For this review, take the finished solid that the model builds, in its own axes (mm). A direction names the side the tool comes from. Give positions to 0.01 mm unless a question says otherwise; leave off trailing zeros. Order: outer loops, then holes, each group sorted by start corner. A loop starts at its lowest first (then second) coordinate and runs counter-clockwise, first axis right, second up. Notation, with made-up numbers: (30.5, 9.25) - (62.5, 9.25) arc R23 ccw to (62.5, 18.25) - close; hole circle Ø2 at (37.25, 19.25). An arc over 180 degrees is marked (long way). Use a Markdown table: item, result. Add a question column.
1) Mouldability with a two-part tool opening along X and no side actions: class faces 3 (the face through (0, 0, 0)), 4 (the face through (9.954, 11.671, 2.504)), 5 (the face through (-2.88, 21.91, 2.5)) as released by +X, released by -X, zero draft, split by the parting line, or undercut.
2) We need section C-C on z = 63.5. Write out the cut boundary in (x, y), then the cut area to 3 significant figures.
3) Clearance check with flat-ended pins moving along their axes: P1, Ø2, axis at x = -9, z = 37.5, coming from the +Y side; P2, Ø10, axis at x = 12.89, y = -12.89, coming from the +Z side; P3, Ø3, axis at y = -7, z = 50.5, coming from the +X side. State where each tip first meets the part, or that it passes through.
4) Wall thickness on L1, parallel to Z at x = 6, y = -15; L2, parallel to Z at x = -11, y = 3.5; L3, parallel to Y at x = -5, z = 59: over which ranges is each line inside the solid? List them lowest first.
5) We need section A-A on x = 0. Write out the cut boundary in (y, z), then the cut area to 3 significant figures.
6) Machinability: for faces 1 (the face through (13.84, -9.86, 2.5)), 2 (the face through (1.93, 8.68, 67.47)), which of the approach directions +Z, -Z, +X, -X, +Y, -Y give a long, thin tool a straight path to every point of the face, cutting with its end or side? Answer none if there is none.
7) We need section D-D on z = 34. Write out the cut boundary in (x, y), then the cut area to 3 significant figures.
```python
from build123d import *

# Parameters (mm, degrees)
SKETCH1_R           = 22.098
BOSS_EXTRUDE1_DEPTH = 5.08
SKETCH2_R           = 14.351
BOSS_EXTRUDE2_DEPTH = 38.1
SKETCH3_R           = 11.811
BOSS_EXTRUDE3_DEPTH = 17.78
SKETCH4_R           = 8.89
BOSS_EXTRUDE4_DEPTH = 13.208
SKETCH6_R           = 3.175
CUT_EXTRUDE1_DEPTH  = 5.08
CIRPATTERN1_COUNT   = 4


with BuildPart() as part:
    # Sketch1 → Boss-Extrude1 (new body)
    with BuildSketch(Plane.XY):
        Circle(SKETCH1_R)
    extrude(amount=BOSS_EXTRUDE1_DEPTH)

    # Sketch2 → Boss-Extrude2 (add)
    with BuildSketch(Plane.XY.offset(5.08)):
        with Locations(Location((0, 0, 0), (0, 0, 180))):
            Circle(SKETCH2_R)
    extrude(amount=BOSS_EXTRUDE2_DEPTH)

    # Sketch3 → Boss-Extrude3 (add)
    with BuildSketch(Plane.XY.offset(43.18)):
        Circle(SKETCH3_R)
    extrude(amount=BOSS_EXTRUDE3_DEPTH)

    # Sketch4 → Boss-Extrude4 (add)
    with BuildSketch(Plane.XY.offset(60.96)):
        with Locations(Location((0, 0, 0), (0, 0, 180))):
            Circle(SKETCH4_R)
    extrude(amount=BOSS_EXTRUDE4_DEPTH)

    # Sketch6 → Cut-Extrude1 (cut)
    with BuildSketch(Plane(origin=(0, 0, 0), x_dir=(-1, 0, 0), z_dir=(0, 0, -1))):
        with Locations((-12.886667534, 12.886667534)):
            Circle(SKETCH6_R)
    cut_extrude1 = extrude(amount=-CUT_EXTRUDE1_DEPTH, mode=Mode.SUBTRACT)

    # CirPattern1: Cut-Extrude1 ×4 about axis
    cirpattern1_axis = Axis((0, 0, 0), (0, 0, 1))
    for i in range(1, CIRPATTERN1_COUNT):
        add(cut_extrude1.rotate(cirpattern1_axis, i * 360 / CIRPATTERN1_COUNT), mode=Mode.SUBTRACT)


solid = part.part
```
Checked values:
| question | item | result |
|---|---|---|
| 1 | face 3 | zero draft |
| 1 | face 4 | undercut |
| 1 | face 5 | split by the parting line |
| 2 | outline | circle Ø17.78 at (0, 0) |
| 2 | area | 248 mm² |
| 3 | P1 | y = 11.91 |
| 3 | P2 | z = 43.18 |
| 3 | P3 | x = 10.45 |
| 4 | L1 | 0 to 5.08 |
| 4 | L2 | 0 to 60.96 |
| 4 | L3 | -10.7 to 10.7 |
| 5 | outline | (-22.1, 0) - (22.1, 0) - (22.1, 5.08) - (14.35, 5.08) - (14.35, 43.18) - (11.81, 43.18) - (11.81, 60.96) - (8.89, 60.96) - (8.89, 74.17) - (-8.89, 74.17) - (-8.89, 60.96) - (-11.81, 60.96) - (-11.81, 43.18) - (-14.35, 43.18) - (-14.35, 5.08) - (-22.1, 5.08) - close |
| 5 | area | 1,970 mm² |
| 6 | face 1 | +Z, -Z |
| 6 | face 2 | +Z |
| 7 | outline | circle Ø28.7 at (0, 0) |
| 7 | area | 647 mm² |
